The model under review builds one solid part; all positions refer to its coordinate system, in mm. Face numbers are marked on the shaded views. A direction names the side the tool comes from. Coordinates: 2 decimals unless noted, no trailing zeros. Write each loop counter-clockwise with the first axis right and the second up, starting at its lowest first coordinate (ties: lowest second). Pieces come first, ordered by that corner, then holes.
1) For P1, Ø5, axis at x = 27, z = 2.5, coming from the +Y side; P2, Ø5, axis at x = 11, y = 11, coming from the -Z side; P3, Ø5, axis at x = 23.5, z = 3.5, coming from the -Y side; P4, Ø3, axis at x = 31.5, z = 4.5, coming from the +Y side, all flat-tipped, find the tip position at first contact; note any pin that passes through.
2) Add section B-B, the plane y = 6. State the section outline as (x, z) points.
3) Machinability: for the marked faces 4 and 5, which of the approach directions +Z, -Z, +X, -X, +Y, -Y give a long, thin tool a straight path to every point of the face, cutting with its end or side? Answer none if there is none.
4) Add section A-A, the plane z = 3.5. State the section outline as (x, y) points, then the cut area to 3 significant figures.
5) Mouldability with a two-part tool opening along Y and no side actions: class the marked faces 1, 2 and 3 as released by +Y, released by -Y, zero draft, split by the parting line, or undercut.
6) For line 1 (Y direction, x = 0, z = 4.5); line 2 (Y direction, x = 12, z = 3.5); line 3 (X direction, y = 29.5, z = 3.5), list the stretches that pass through material, from the lowest coordinate up.
7) Add section C-C, the plane x = 33.5. State the section outline as (y, z) points, then the cut area to 3 significant figures.
from build123d import *

# Parameters (mm, degrees)
SALIENTE_EXTRUIR2_DEPTH = 10
CROQUIS2_R              = 2
CORTAR_EXTRUIR1_DEPTH   = 90.57535888
SALIENTE_EXTRUIR3_START = -5
SALIENTE_EXTRUIR3_DEPTH = 5
CROQUIS4_R              = 3.5
CORTAR_EXTRUIR2_DEPTH   = 10


with BuildPart() as part:
    # Croquis1 → Saliente-Extruir2 (new body)
    with BuildSketch(Plane.XY):
        with BuildLine():
            Line((44.628418222, 52.139361077), (0, 4.5))
            ThreePointArc((0, 4.5), (-1.767766953, 0.232233047), (2.5, 2))
            Line((2.5, 2), (54.328418222, 42.439361077))
            ThreePointArc((54.328418222, 42.439361077), (61.187353999, 58.998296855), (44.628418222, 52.139361077))
        make_face()
        with BuildLine():
            Line((53.992751033, 43.445838918), (2.255737897, 3.077797078))
            ThreePointArc((2.255737897, 3.077797078), (1.78485494, 3.750512166), (1.121414308, 4.234374622))
            Line((1.121414308, 4.234374622), (45.636989072, 51.753279039))
            ThreePointArc((45.636989072, 51.753279039), (60.462381656, 58.309003902), (53.992751033, 43.445838918))
        make_face(mode=Mode.SUBTRACT)
    extrude(amount=SALIENTE_EXTRUIR2_DEPTH)

    # Croquis2 → Cortar-Extruir1 (cut, through all)
    with BuildSketch(Plane.XY.offset(10)):
        with Locations((0, 2)):
            Circle(CROQUIS2_R)
    extrude(amount=-CORTAR_EXTRUIR1_DEPTH, mode=Mode.SUBTRACT)

    # Croquis3 → Saliente-Extruir3 (add)
    with BuildSketch(Plane.XY.offset(10).offset(SALIENTE_EXTRUIR3_START)):
        with BuildLine():
            Line((53.992751033, 43.445838918), (2.255737897, 3.077797078))
            ThreePointArc((2.255737897, 3.077797078), (1.78485494, 3.750512166), (1.121414308, 4.234374622))
            Line((1.121414308, 4.234374622), (45.636989072, 51.753279039))
            ThreePointArc((45.636989072, 51.753279039), (60.462381656, 58.309003902), (53.992751033, 43.445838918))
        make_face()
    extrude(amount=SALIENTE_EXTRUIR3_DEPTH)

    # Croquis4 → Cortar-Extruir2 (cut)
    with BuildSketch(Plane(origin=(0, 0, 5), x_dir=(-1, 0, 0), z_dir=(0, 0, -1))):
        with Locations((-54.328418222, 52.139361077)):
            Circle(CROQUIS4_R)
    extrude(amount=-CORTAR_EXTRUIR2_DEPTH, mode=Mode.SUBTRACT)


solid = part.part
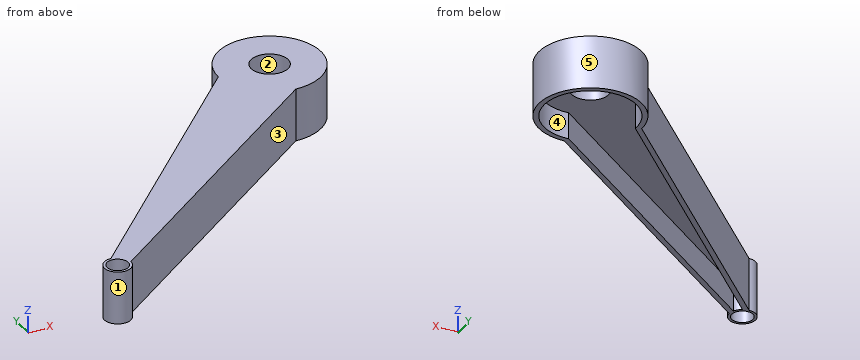
Geometry results:
1. P1: stops at y = 35.99
1. P2: stops at z = 0
1. P3: stops at y = 16.43
1. P4: stops at y = 39.73
2. outline: (1.41, 0) - (2.78, 0) - (2.78, 5) - (6, 5) - (6, 0) - (7.63, 0) - (7.63, 10) - (1.41, 10) - close
3. face 4: -Z
3. face 5: +Z, -Z
4. outline: (0, 4.5) arc R2.5 ccw (long way) to (2.5, 2) - (54.33, 42.44) arc R9.7 ccw (long way) to (44.63, 52.14) - close; hole circle Ø4 at (0, 2); hole (1.12, 4.23) arc R2.5 cw to (2.26, 3.08) - (53.99, 43.45) arc R8.7 ccw (long way) to (45.64, 51.75) - close
4. area: 182 mm2
5. face 1: split by the parting line
5. face 2: undercut
5. face 3: released by -Y
6. line 1: y = -0.5 to 0, 4 to 4.5
6. line 2: y = 9.41 to 10.68, 15.85 to 17.31
6. line 3: x = 23.42 to 24.79, 36.12 to 37.74
7. outline: (26.19, 0) - (27.46, 0) - (27.46, 5) - (38.8, 5) - (38.8, 0) - (40.26, 0) - (40.26, 10) - (26.19, 10) - close
7. area: 84.0 mm2
